Source: CAD feature listing. Evaluate the final solid. Frame: model axes, mm. Face numbers are marked on the shaded views. A direction names the side the tool comes from. Round coordinates to 2 decimals unless told otherwise and drop trailing zeros. Write each loop counter-clockwise with the first axis right and the second up, starting at its lowest first coordinate (ties: lowest second). Pieces come first, ordered by that corner, then holes. Notation, with made-up numbers: M -33.5,-17 L 6.5,-17 A9 cw 6.5,-12 Z; hole C 36,67.5 d6. An arc over 180 degrees is marked long. Put each result on its own line as item: value. Start each with the question number.
```python
from build123d import *

# Parameters (mm, degrees)
SKETCH1_W                 = 150
SKETCH1_H                 = 54.5
BOSS_EXTRUDE1_DEPTH       = 5
SKETCH2_W                 = 5
SKETCH2_H                 = 54.5
BOSS_EXTRUDE2_DEPTH       = 8
F_8_CLEARANCE_HOLE1_D     = 4.4958
F_8_CLEARANCE_HOLE1_DEPTH = 17
F_8_CLEARANCE_HOLE1_TIP   = 1.350674586
SKETCH7_W                 = 5
SKETCH7_H                 = 54.5
BOSS_EXTRUDE3_DEPTH       = 43
SKETCH8_R                 = 4.25
CUT_EXTRUDE1_DEPTH        = 4
RIB1_REACH                = 120.085
SKETCH10_WALL_W           = 279.571445908
SKETCH10_WALL_H           = 10
RIB3_REACH                = 120.085
SKETCH12_WALL_W           = 279.571445908
SKETCH12_WALL_H           = 10
SKETCH13_W                = 8
SKETCH13_H                = 2
BOSS_EXTRUDE4_DEPTH       = 5
SKETCH14_R                = 2
CUT_EXTRUDE2_DEPTH        = 2
SKETCH15_R                = 3.5
CUT_EXTRUDE3_DEPTH        = 1
SKETCH16_W                = 3
SKETCH16_H                = 12
CUT_EXTRUDE4_DEPTH        = 5
F_8_CLEARANCE_HOLE2_D     = 4.4958
F_8_CLEARANCE_HOLE2_DEPTH = 17
F_8_CLEARANCE_HOLE2_TIP   = 1.350674586


with BuildPart() as part:
    # Sketch1 → Boss-Extrude1 (new body)
    with BuildSketch(Plane(origin=(0, 0, 0), x_dir=(1, 0, 0), z_dir=(0, 1, 0))):
        with Locations((-18.112463826, -1.689393939)):
            Rectangle(SKETCH1_W, SKETCH1_H)
    extrude(amount=BOSS_EXTRUDE1_DEPTH)

    # Sketch2 → Boss-Extrude2 (add)
    with BuildSketch(Plane(origin=(0, 5, 0), x_dir=(1, 0, 0), z_dir=(0, 1, 0))):
        with Locations((-90.612463826, -1.689393939)):
            Rectangle(SKETCH2_W, SKETCH2_H)
    extrude(amount=BOSS_EXTRUDE2_DEPTH)

    # #8 Clearance Hole1
    with Locations(Plane(origin=(-93.112463826, 9.2, -15.560606061), x_dir=(0, 0, -1), z_dir=(-1, 0, 0))):
        with Locations((0, 0), (-17.25, 0), (-34.5, 0)):
            Hole(F_8_CLEARANCE_HOLE1_D / 2, depth=F_8_CLEARANCE_HOLE1_DEPTH)
            with Locations((0, 0, -(F_8_CLEARANCE_HOLE1_DEPTH + F_8_CLEARANCE_HOLE1_TIP / 2))):  # 118° drill point
                Cone(0, F_8_CLEARANCE_HOLE1_D / 2, F_8_CLEARANCE_HOLE1_TIP, mode=Mode.SUBTRACT)

    # Sketch7 → Boss-Extrude3 (add)
    with BuildSketch(Plane(origin=(0, 5, 0), x_dir=(1, 0, 0), z_dir=(0, 1, 0))):
        with Locations((54.387536174, -1.689393939)):
            Rectangle(SKETCH7_W, SKETCH7_H)
    extrude(amount=BOSS_EXTRUDE3_DEPTH)

    # Sketch8 → Cut-Extrude1 (cut)
    with BuildSketch(Plane.ZY.offset(-51.887536174)):
        with Locations((-15.560606061, 43)):
            Circle(SKETCH8_R)
        with Locations((18.939393939, 43)):
            Circle(SKETCH8_R)
    extrude(amount=-CUT_EXTRUDE1_DEPTH, mode=Mode.SUBTRACT)

    # Sketch10 wall → Rib1 (add, up to next)
    with BuildSketch(Plane(origin=(39.387536174, 21.5, -25.560606061), x_dir=(-0.603857687995, -0.797092148154, 0), z_dir=(-0.797092148154, 0.603857687995, 0)), mode=Mode.PRIVATE) as rib1_sk1:
        with Locations((0, 5)):
            Rectangle(SKETCH10_WALL_W, SKETCH10_WALL_H)
    rib1_tool1 = extrude(rib1_sk1.sketch, amount=-RIB1_REACH, mode=Mode.PRIVATE) - part.part
    add(rib1_tool1.solids().sort_by_distance((39.387536174, 21.5, -25.560606061))[0])

    # Sketch12 wall → Rib3 (add, up to next)
    with BuildSketch(Plane(origin=(39.387536174, 21.5, 28.939393939), x_dir=(-0.603857687995, -0.797092148154, 0), z_dir=(0.797092148154, -0.603857687995, 0)), mode=Mode.PRIVATE) as rib3_sk1:
        with Locations((0, 5)):
            Rectangle(SKETCH12_WALL_W, SKETCH12_WALL_H)
    rib3_tool1 = extrude(rib3_sk1.sketch, amount=RIB3_REACH, mode=Mode.PRIVATE) - part.part
    add(rib3_tool1.solids().sort_by_distance((39.387536174, 21.5, 28.939393939))[0])

    # Sketch13 → Boss-Extrude4 (add)
    with BuildSketch(Plane.ZY.offset(-51.887536174)):
        with Locations((1.689393939, 37)):
            Rectangle(SKETCH13_W, SKETCH13_H)
    extrude(amount=BOSS_EXTRUDE4_DEPTH)

    # Sketch14 → Cut-Extrude2 (cut)
    with BuildSketch(Plane(origin=(0, 38, 0), x_dir=(1, 0, 0), z_dir=(0, 1, 0))):
        with Locations(Location((49.387536174, -1.689393939, 0), (0, 0, 270))):
            Circle(SKETCH14_R)
    extrude(amount=-CUT_EXTRUDE2_DEPTH, mode=Mode.SUBTRACT)

    # Sketch15 → Cut-Extrude3 (cut)
    with BuildSketch(Plane.ZY.offset(-55.887536174)):
        with Locations((-15.560606061, 43)):
            Circle(SKETCH15_R)
        with Locations((18.939393939, 43)):
            Circle(SKETCH15_R)
    extrude(amount=-CUT_EXTRUDE3_DEPTH, mode=Mode.SUBTRACT)

    # Sketch16 → Cut-Extrude4 (cut)
    with BuildSketch(Plane(origin=(0, 5, 0), x_dir=(1, 0, 0), z_dir=(0, 1, 0))):
        with Locations((0.387536174, 15.560606061)):
            Rectangle(SKETCH16_W, SKETCH16_H)
        with Locations((0.387536174, -18.939393939)):
            Rectangle(SKETCH16_W, SKETCH16_H)
    extrude(amount=-CUT_EXTRUDE4_DEPTH, mode=Mode.SUBTRACT)

    # #8 Clearance Hole2
    with Locations(Plane(origin=(-3.112463826, 5, 1.689393939), x_dir=(0, 0, 1), z_dir=(0, 1, 0))):
        with Locations((0, 0), (13.625, -30), (-13.625, -30)):
            Hole(F_8_CLEARANCE_HOLE2_D / 2, depth=F_8_CLEARANCE_HOLE2_DEPTH)
            with Locations((0, 0, -(F_8_CLEARANCE_HOLE2_DEPTH + F_8_CLEARANCE_HOLE2_TIP / 2))):  # 118° drill point
                Cone(0, F_8_CLEARANCE_HOLE2_D / 2, F_8_CLEARANCE_HOLE2_TIP, mode=Mode.SUBTRACT)


solid = part.part
```
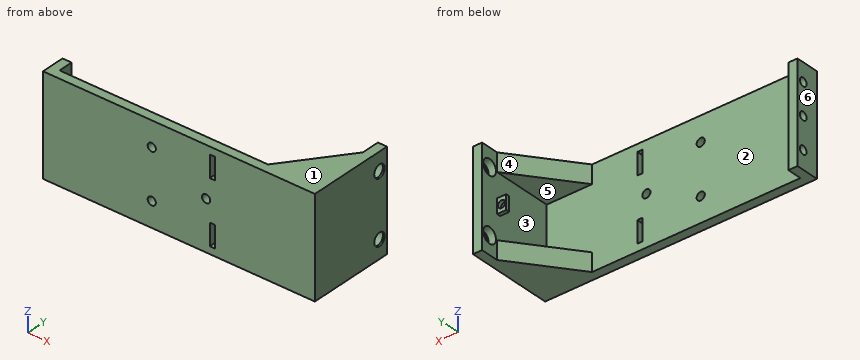
(1) Ray query, line 1 along Z through (x, y) = (-91, 9); line 2 along Z through (x, y) = (47.5, 26.5); line 3 along X through (y, z) = (11, 5). Return the intervals inside material, ascending.
(2) Section query D-D (y = 19). Return loops of the section in (x, z).
(3) Pull-direction query (Z, two-part tool) for the marked faces 1, 2, 3 and 4; classes: +Z half, -Z half, draft (parallel to the pull), parting line (faces both ways), or undercut.
(4) Section query C-C (y = 9.2). Return loops of the section in (x, z).
(5) Section query A-A (y = 43). Return loops of the section in (x, z), and give its area (4 significant figures).
(6) Access query for the marked faces 5 and 6. Directions: +Z, -Z, +X, -X, +Y, -Y. A direction counts if a zero-diameter tool reaches every point of the face in a straight line with its end or side. Return the directions, or none.
(7) Contact query for flat-ended pins moving along their axis: P1, Ø3, axis at x = -69, z = -12, coming from the +Y side; P2, Ø1, axis at y = 37, z = 3, coming from the -X side; P3, Ø10, axis at y = 37.5, z = -16.5, coming from the -X side. Output: stop coordinate, or through.
(8) Section query B-B (x = 32). Return loops of the section in (y, z).
Entries:
1. line 1: -25.56 to -17.8, -13.32 to -0.55, 3.93 to 16.7, 21.18 to 28.94
1. line 2: -25.56 to -15.56, 18.94 to 28.94
1. line 3: -93.11 to -88.11, 51.89 to 56.89
2. outline: M 37.49,-25.56 L 56.89,-25.56 L 56.89,28.94 L 37.49,28.94 L 37.49,18.94 L 51.89,18.94 L 51.89,-15.56 L 37.49,-15.56 Z
3. face 1: +Z half
3. face 2: undercut
3. face 3: undercut
3. face 4: draft
4. outline: M -93.11,-25.56 L -88.11,-25.56 L -88.11,-17.81 L -93.11,-17.81 Z; M -93.11,-13.31 L -88.11,-13.31 L -88.11,-0.56 L -93.11,-0.56 Z; M -93.11,3.94 L -88.11,3.94 L -88.11,16.69 L -93.11,16.69 Z; M -93.11,21.19 L -88.11,21.19 L -88.11,28.94 L -93.11,28.94 Z; M 30.07,-25.56 L 56.89,-25.56 L 56.89,28.94 L 30.07,28.94 L 30.07,18.94 L 51.89,18.94 L 51.89,-15.56 L 30.07,-15.56 Z
5. outline: M 51.89,-25.56 L 56.89,-25.56 L 56.89,-19.06 L 55.89,-19.06 L 55.89,-19.81 L 51.89,-19.81 Z; M 51.89,-11.31 L 55.89,-11.31 L 55.89,-12.06 L 56.89,-12.06 L 56.89,15.44 L 55.89,15.44 L 55.89,14.69 L 51.89,14.69 Z; M 51.89,23.19 L 55.89,23.19 L 55.89,22.44 L 56.89,22.44 L 56.89,28.94 L 51.89,28.94 Z
5. area: 190.5 mm2
6. face 5: +Y
6. face 6: +Z, -Z, -X, +Y, -Y
7. P1: y = 5
7. P2: x = 46.89
7. P3: x = 47.72
8. outline: M 0,-25.56 L 11.75,-25.56 L 11.75,-15.56 L 5,-15.56 L 5,18.94 L 11.75,18.94 L 11.75,28.94 L 0,28.94 Z
